Work out the finished part from the listing and answer in its coordinate system (mm). Face numbers are marked on the shaded views. Coordinates: 2 decimals unless noted, no trailing zeros. Order: outer loops, then holes, each group sorted by start corner. A loop starts at its lowest first (then second) coordinate and runs counter-clockwise, first axis right, second up.
1. Determine the mould class of the marked faces 1, 2, 3 and 4 for opening direction X: +X half, -X half, draft (parallel to the pull), parting line (faces both ways), or undercut.
2. The part is cut by section A-A, the plane x = 0. Give the vertices of the cut face in (y, z), then the cut area to 3 significant figures.
3. Find the intervals of material crossed by probe 1 along X at (y, z) = (17, 6); probe 2 along Y at (x, z) = (16, 4); probe 3 along X at (y, z) = (15, 3.25), in increasing order.
4. A flat-ended cylindrical pin translates along its axis: pin 1 Ø1.8 at (x, y) = (16, 16) entering from -Z. Find the tip coordinate at first contact, or state that the pin passes through.
5. The part is cut by section C-C, the plane z = 6.5. Give the vertices of the cut face in (x, y).
6. The part is cut by section D-D, the plane y = 16. Give the vertices of the cut face in (x, z), then the cut area to 3 significant figures.
```python
from build123d import *

# Parameters (mm, degrees)
SKETCH_1_W          = 40
SKETCH_1_H          = 40
EXTRUDE_1_DEPTH     = 10
SKETCH_2_R          = 19
CUT_EXTRUDE_1_DEPTH = 31
SKETCH_3_R          = 1.5
CUT_EXTRUDE_2_DEPTH = 31


with BuildPart() as part:
    # 草圖1 → 填料-伸長1 (new body)
    with BuildSketch(Plane.XY):
        Rectangle(SKETCH_1_W, SKETCH_1_H)
    extrude(amount=EXTRUDE_1_DEPTH)

    # 草圖2 → 除料-伸長1 (cut, through all)
    with BuildSketch(Plane.XY.offset(10)):
        Circle(SKETCH_2_R)
    extrude(amount=-CUT_EXTRUDE_1_DEPTH, mode=Mode.SUBTRACT)

    # 草圖3 → 除料-伸長2 (cut, through all)
    with BuildSketch(Plane.XY.offset(10)):
        with Locations((-16, 16)):
            Circle(SKETCH_3_R)
        with Locations((-16, -16)):
            Circle(SKETCH_3_R)
        with Locations((16, -16)):
            Circle(SKETCH_3_R)
        with Locations((16, 16)):
            Circle(SKETCH_3_R)
    extrude(amount=-CUT_EXTRUDE_2_DEPTH, mode=Mode.SUBTRACT)


solid = part.part
```
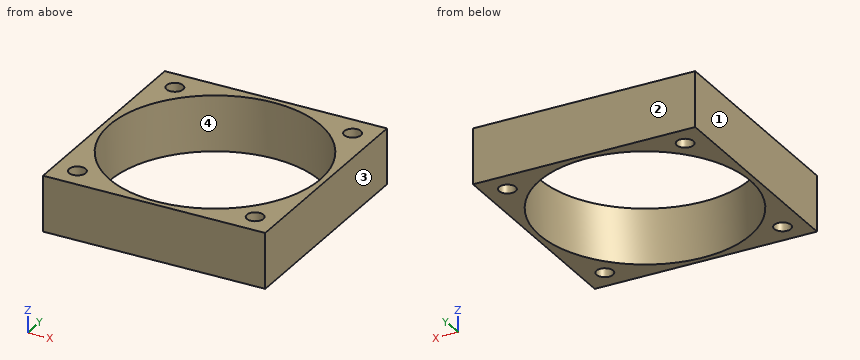
Geometry says:
1. face 1: -X half
1. face 2: draft
1. face 3: +X half
1. face 4: undercut
2. outline: (-20, 0) - (-19, 0) - (-19, 10) - (-20, 10) - close; (19, 0) - (20, 0) - (20, 10) - (19, 10) - close
2. area: 20.0 mm2
3. probe 1: x = -20 to -17.12, -14.88 to -8.49, 8.49 to 14.88, 17.12 to 20
3. probe 2: y = -20 to -17.5, -14.5 to -10.25, 10.25 to 14.5, 17.5 to 20
3. probe 3: x = -20 to -17.12, -14.88 to -11.66, 11.66 to 14.88, 17.12 to 20
4. pin 1: passes through
5. outline: (-20, -20) - (20, -20) - (20, 20) - (-20, 20) - close; hole circle Ø38 at (0, 0); hole circle Ø3 at (-16, -16); hole circle Ø3 at (-16, 16); hole circle Ø3 at (16, -16); hole circle Ø3 at (16, 16)
6. outline: (-20, 0) - (-17.5, 0) - (-17.5, 10) - (-20, 10) - close; (-14.5, 0) - (-10.25, 0) - (-10.25, 10) - (-14.5, 10) - close; (10.25, 0) - (14.5, 0) - (14.5, 10) - (10.25, 10) - close; (17.5, 0) - (20, 0) - (20, 10) - (17.5, 10) - close
6. area: 135 mm2
